Verification items for the finished model (mm, model axes). Face numbers are marked on the shaded views. A direction names the side the tool comes from. Give positions to 0.01 mm unless a question says otherwise; leave off trailing zeros. Loops run counter-clockwise (first coordinate to the right, second up) from the corner with the lowest first, then second, coordinate; pieces in that order, holes last. Notation, with made-up numbers: (-7.5, 67.25) - (-0.5, 67.25) arc R21 ccw to (-0.5, 103.25) - close; hole circle Ø10 at (38, 77). An arc over 180 degrees is marked (long way). Use one line per item in the form item = value.
```python
from build123d import *

# Parameters (mm, degrees)
EXTRUDE_1_DEPTH      = 10
EXTRUDE_1_DEPTH_BACK = 20
EXTRUDE_2_DEPTH      = 20
EXTRUDE_3_DEPTH      = 10
SKETCH_5_W           = 84
SKETCH_5_H           = 24
CUT_EXTRUDE_1_DEPTH  = 17
SKETCH_4_R           = 2.5
SKETCH_4_R_2         = 1.1
CUT_EXTRUDE_2_DEPTH  = 17
SKETCH_6_R           = 2.210367197
CUT_EXTRUDE_3_DEPTH  = 8
SKETCH_7_W           = 3
SKETCH_7_H           = 52.500208742
EXTRUDE_4_DEPTH      = 25
SKETCH_8_R           = 1.095411725
SKETCH_8_W           = 32
SKETCH_8_H           = 20.937005418
CUT_EXTRUDE_6_DEPTH  = 5


with BuildPart() as part:
    # Sketch 1 → Extrude 1 (new body, two sides)
    with BuildSketch(Plane(origin=(0, 0, 0), x_dir=(1, 0, 0), z_dir=(0, 1, 0))) as extrude_1_sk:
        with BuildLine():
            ThreePointArc((-4.68866799, 114.767541166), (0.26262686, 59.767541166), (-4.68866799, 4.767541166))
            Line((-4.68866799, 4.767541166), (-7.68866799, 4.767541166))
            ThreePointArc((-7.68866799, 4.767541166), (-2.68866799, 59.767541166), (-7.68866799, 114.767541166))
            Line((-7.68866799, 114.767541166), (-4.68866799, 114.767541166))
        make_face()
    extrude(amount=EXTRUDE_1_DEPTH)
    extrude(extrude_1_sk.sketch, amount=-EXTRUDE_1_DEPTH_BACK)



with BuildPart() as body_2:
    # Sketch 1_3 → Extrude 2 (new body)
    with BuildSketch(Plane(origin=(0, 0, 0), x_dir=(1, 0, 0), z_dir=(0, 1, 0))):
        with BuildLine():
            Line((11.598251721, 104.872295398), (-3.058464061, 104.872295398))
            ThreePointArc((-3.058464061, 104.872295398), (0.262608655, 59.873432048), (-3.027517025, 14.872295398))
            Line((-3.027517025, 14.872295398), (11.598251721, 14.872295398))
            Line((11.598251721, 14.872295398), (11.598251721, 104.872295398))
        make_face()
    extrude(amount=-EXTRUDE_2_DEPTH)


with BuildPart() as part_1:
    add(part.part)

    add(body_2.part)  # Extrude 3 merges body 2
    # Sketch 1_4 → Extrude 3 (add)
    with BuildSketch(Plane(origin=(0, 0, 0), x_dir=(1, 0, 0), z_dir=(0, 1, 0))):
        with BuildLine():
            Line((11.598251721, 104.872295398), (-3.058464061, 104.872295398))
            ThreePointArc((-3.058464061, 104.872295398), (0.262608655, 59.873432048), (-3.027517025, 14.872295398))
            Line((-3.027517025, 14.872295398), (11.598251721, 14.872295398))
            Line((11.598251721, 14.872295398), (11.598251721, 104.872295398))
        make_face()
    extrude(amount=EXTRUDE_3_DEPTH)

    # Sketch 5 → Cut-Extrude 1 (cut)
    with BuildSketch(Plane(origin=(-8.401748279, 0, 0), x_dir=(0, 0, -1), z_dir=(1, 0, 0))):
        with Locations((59.767541166, -5.056638817)):
            Rectangle(SKETCH_5_W, SKETCH_5_H)
    extrude(amount=CUT_EXTRUDE_1_DEPTH, mode=Mode.SUBTRACT)

    # Sketch 4 → Cut-Extrude 2 (cut)
    with BuildSketch(Plane(origin=(11.598251721, 0, 0), x_dir=(0, 0, -1), z_dir=(1, 0, 0))):
        with Locations((30.172295398, 4.863328118)):
            Circle(SKETCH_4_R)
        with Locations((89.572295398, 4.863328118)):
            Circle(SKETCH_4_R)
        with Locations((89.572295398, -12.936671882)):
            Circle(SKETCH_4_R)
        with Locations((30.172295398, -12.936671882)):
            Circle(SKETCH_4_R)
        with Locations((21.172295398, -12.936671882)):
            Circle(SKETCH_4_R_2)
        with Locations((21.172295398, 4.863328118)):
            Circle(SKETCH_4_R_2)
        with Locations((98.572295398, 4.863328118)):
            Circle(SKETCH_4_R_2)
        with Locations((98.572295398, -12.936671882)):
            Circle(SKETCH_4_R_2)
    extrude(amount=-CUT_EXTRUDE_2_DEPTH, mode=Mode.SUBTRACT)

    # Sketch 6 → Cut-Extrude 3 (cut)
    with BuildSketch(Plane(origin=(-8.401748279, 0, 0), x_dir=(0, 0, -1), z_dir=(1, 0, 0))):
        with Locations(Location((9.665216794, -5.258703912, 0), (0, 0, 180))):  # turned: the seam where the file's is
            Circle(SKETCH_6_R)
        with Locations(Location((110.079374003, -5.258703912, 0), (0, 0, 180))):  # turned: the seam where the file's is
            Circle(SKETCH_6_R)
    extrude(amount=CUT_EXTRUDE_3_DEPTH, mode=Mode.SUBTRACT)

    # Sketch 7 → Extrude 4 (add)
    with BuildSketch(Plane.XZ.offset(20)):
        with Locations((7.115575895, -59.872295398)):
            Rectangle(SKETCH_7_W, SKETCH_7_H)
    extrude(amount=EXTRUDE_4_DEPTH)

    # Sketch 8 → Cut-Extrude 6 (cut)
    with BuildSketch(Plane(origin=(8.615575895, 0, 0), x_dir=(0, 0, -1), z_dir=(1, 0, 0))):
        with Locations((38.872295398, -24.471390048)):
            Circle(SKETCH_8_R)
        with Locations((38.872295398, -41.471390048)):
            Circle(SKETCH_8_R)
        with Locations((80.872295398, -41.471390048)):
            Circle(SKETCH_8_R)
        with Locations((80.872295398, -24.471390048)):
            Circle(SKETCH_8_R)
        with Locations((59.872295398, -34.531497291)):
            Rectangle(SKETCH_8_W, SKETCH_8_H)
    extrude(amount=-CUT_EXTRUDE_6_DEPTH, mode=Mode.SUBTRACT)


solid = part_1.part
```
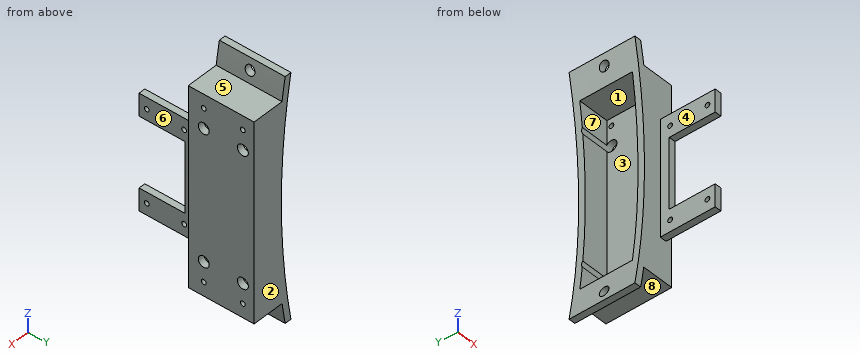
1. Section check C-C, the plane x = 10.25. State how many separate pieces and enclosed holes the cut face has, then the cut area to 3 significant figures.
Result set:
separate_pieces = 1
enclosed_holes = 8
area = 2,610 mm²
2. Section check A-A, the plane x = -1. Record the cut outline in (y, z), then the cut area to 3 significant figures.
Result set:
outline = (-20, -104.87) - (10, -104.87) - (10, -14.87) - (-20, -14.87) - close; hole (-17.06, -101.77) - (6.94, -101.77) - (6.94, -90.96) arc R2.5 ccw to (6.94, -88.19) - (6.94, -31.56) arc R2.5 ccw to (6.94, -28.79) - (6.94, -17.77) - (-17.06, -17.77) - close
area = 682 mm²
3. Section check D-D, the plane z = -57.5. Record the cut outline in (x, y).
Result set:
outline = (-2.7, -20) - (5.62, -20) - (5.62, -24.06) - (8.62, -24.06) - (8.62, -20) - (11.6, -20) - (11.6, 10) - (-2.7, 10) - (-2.7, 6.94) - (8.6, 6.94) - (8.6, -17.06) - (-2.7, -17.06) - close
4. Section check B-B, the plane y = -39. Record the cut outline in (x, z), then the cut area to 3 significant figures.
Result set:
outline = (5.62, -86.12) - (8.62, -86.12) - (8.62, -75.87) - (5.62, -75.87) - close; (5.62, -43.87) - (8.62, -43.87) - (8.62, -33.62) - (5.62, -33.62) - close
area = 61.5 mm²
5. Scan lines: probe 1 along Z at (x, y) = (7.25, -30.5); probe 2 along Y at (x, z) = (8.5, -101.5); probe 3 along Z at (x, y) = (1.75, -5). Record each from-to range of solid material in increasing order.
Result set:
probe_1 = -86.12 to -75.87, -43.87 to -33.62
probe_2 = -20 to -17.06, 6.94 to 10
probe_3 = -104.87 to -101.77, -17.77 to -14.87
6. Tool access check on the marked faces 5, 6, 7 and 8. Record the directions out of +Z, -Z, +X, -X, +Y, -Y that give a thin tool (end or side, any length) a straight path to the whole face; none if there is none.
Result set:
face_5 = +Z, +X, +Y, -Y
face_6 = +Z, -Z, +X, -Y
face_7 = -X
face_8 = -Z, +X, +Y, -Y
7. Draft check along Y on the marked faces 1, 2, 3 and 4. Enter one of: released by +Y, released by -Y, zero draft, split by the parting line, or undercut.
Result set:
face_1 = undercut
face_2 = released by +Y
face_3 = undercut
face_4 = zero draft
8. Depth check by flat-ended pin: pin 1 Ø2.5 at (x, y) = (7.5, -27) entering from -Z; pin 2 Ø10 at (x, z) = (0.5, -58.5) entering from -Y; pin 3 Ø0.9 at (x, y) = (7, -37.5) entering from +Z. Enter the tip coordinate at first touch or a pass-through.
Result set:
pin_1 = -86.12
pin_2 = -20
pin_3 = -33.62
